```python
from build123d import *

# Parameters (mm, degrees)
ESQUISSE1_R             = 2
ESQUISSE1_R_2           = 1.5
BOSS_EXTRU_1_DEPTH      = 3
ESQUISSE3_R             = 7.5
BOSS_EXTRU_2_DEPTH      = 6
ESQUISSE4_R             = 3.875
ENL_V_MAT_EXTRU_1_DEPTH = 1
ESQUISSE5_R             = 2.375
ENL_V_MAT_EXTRU_2_DEPTH = 4


with BuildPart() as part:
    # Esquisse1 → Boss.-Extru.1 (new body)
    with BuildSketch(Plane.XY):
        Polygon((0, 50), (-100, 50), (-100, 0), (-61.381557247, 0), (-61.381557247, -45.5212086), (-25, -45.5212086), (-25, -80), (25, -80), (25, -45.5212086), (61.381557247, -45.5212086), (61.381557247, 0), (100, 0), (100, 50), align=None)
        with Locations((0, 20)):
            Circle(ESQUISSE1_R, mode=Mode.SUBTRACT)
        with Locations((0, -20)):
            Circle(ESQUISSE1_R, mode=Mode.SUBTRACT)
        with Locations((0, 40)):
            Circle(ESQUISSE1_R, mode=Mode.SUBTRACT)
        with Locations((-20, -55)):
            Circle(ESQUISSE1_R_2, mode=Mode.SUBTRACT)
        with Locations((20, -55)):
            Circle(ESQUISSE1_R_2, mode=Mode.SUBTRACT)
        with Locations((20, -75)):
            Circle(ESQUISSE1_R_2, mode=Mode.SUBTRACT)
        with Locations((-20, -75)):
            Circle(ESQUISSE1_R_2, mode=Mode.SUBTRACT)
        with Locations((-95, 45)):
            Circle(ESQUISSE1_R_2, mode=Mode.SUBTRACT)
        with Locations((-75, 45)):
            Circle(ESQUISSE1_R_2, mode=Mode.SUBTRACT)
        with Locations((-75, 5)):
            Circle(ESQUISSE1_R_2, mode=Mode.SUBTRACT)
        with Locations((-95, 5)):
            Circle(ESQUISSE1_R_2, mode=Mode.SUBTRACT)
        with Locations((75, 5)):
            Circle(ESQUISSE1_R_2, mode=Mode.SUBTRACT)
        with Locations((95, 5)):
            Circle(ESQUISSE1_R_2, mode=Mode.SUBTRACT)
        with Locations((75, 45)):
            Circle(ESQUISSE1_R_2, mode=Mode.SUBTRACT)
        with Locations((95, 45)):
            Circle(ESQUISSE1_R_2, mode=Mode.SUBTRACT)
        with Locations((56.381557247, -40.5212086)):
            Circle(ESQUISSE1_R, mode=Mode.SUBTRACT)
        with Locations((-56.381557247, -40.5212086)):
            Circle(ESQUISSE1_R, mode=Mode.SUBTRACT)
    extrude(amount=BOSS_EXTRU_1_DEPTH)

    # Esquisse3 → Boss.-Extru.2 (add)
    with BuildSketch(Plane(origin=(0, 0, 0), x_dir=(-1, 0, 0), z_dir=(0, 0, -1))):
        with Locations((0, 20)):
            Circle(ESQUISSE3_R)
        with Locations((56.381557247, -40.5212086)):
            Circle(ESQUISSE3_R)
    extrude(amount=-BOSS_EXTRU_2_DEPTH)

    # Esquisse4 → Enlèv. mat.-Extru.1 (cut)
    with BuildSketch(Plane.XY.offset(6)):
        with Locations((-56.381557247, -40.5212086)):
            Circle(ESQUISSE4_R)
        with Locations((0, 20)):
            Circle(ESQUISSE4_R)
    extrude(amount=-ENL_V_MAT_EXTRU_1_DEPTH, mode=Mode.SUBTRACT)

    # Esquisse5 → Enlèv. mat.-Extru.2 (cut)
    with BuildSketch(Plane.XY.offset(5)):
        with Locations((-56.381557247, -40.5212086)):
            Circle(ESQUISSE5_R)
        with Locations((0, 20)):
            Circle(ESQUISSE5_R)
    extrude(amount=-ENL_V_MAT_EXTRU_2_DEPTH, mode=Mode.SUBTRACT)


solid = part.part
```
Verification items for the finished model (mm, model axes). A direction names the side the tool comes from. Give positions to 0.01 mm unless a question says otherwise; leave off trailing zeros. Order: outer loops, then holes, each group sorted by start corner. A loop starts at its lowest first (then second) coordinate and runs counter-clockwise, first axis right, second up. Notation, with made-up numbers: M 58.25,33 L 84.25,33 A20 ccw 84.25,48 Z; hole C 24,-34.5 d5. An arc over 180 degrees is marked long. Answer in a Markdown table with one row per item. Add a question column.
Item 1: Section check D-D, the plane y = -20. Enter the section's corners in (x, z).
Item 2: Section check B-B, the plane y = 20. Enter the section's corners in (x, z) (3 decimals).
Item 3: Gauge pin test, flat ends, axial feed: pin 1 (2.5 mm diameter, centred on y = -58, z = 1.5, fed in from -X); pin 2 (4 mm diameter, centred on x = 0, y = 20, fed in from +Z); pin 3 (4 mm diameter, centred on x = -20, y = -55, fed in from +Z); pin 4 (3 mm diameter, centred on x = 0, y = -20, fed in from +Z). Record the tip position at first contact, or that the pin passes through.
Item 4: Section check A-A, the plane y = 40. Enter the section's corners in (x, z).
Item 5: Mould release check, pull along Y, two halves, no side actions. Record for faces 3 (the cylindrical face through (0.976, 27.436, 4.479)), 4 (the cylindrical face through (54.907, -39.17, 1.479)), 5 (the cylindrical face through (0, 38, 1)), 6 (the flat face through (-3, 17, 6)): released by +Y, released by -Y, zero draft, split by the parting line, or undercut.
Item 6: Scan lines: probe 1 along Y at (x, z) = (-95, 1.45); probe 2 along Y at (x, z) = (20, 1.9); probe 3 along X at (y, z) = (4, 0.55). Record each from-to range of solid material in increasing order. Write a range as from..to.
Item 7: Section check C-C, the plane x = 46.5. Enter the section's corners in (y, z).
Item 8: Tool access check on faces 1 (the cylindrical face through (0, -18, 1)), 2 (the flat face through (0, 20, 1)). Record the directions out of +Z, -Z, +X, -X, +Y, -Y that give a thin tool (end or side, any length) a straight path to the whole face; none if there is none.
Filled sheet:
| question | item | result |
|---|---|---|
| 1 | outline | M -61.38,0 L -2,0 L -2,3 L -61.38,3 Z; M 2,0 L 61.38,0 L 61.38,3 L 2,3 Z |
| 2 | outline | M -100,0 L 100,0 L 100,3 L 7.5,3 L 7.5,6 L 3.875,6 L 3.875,5 L 2.375,5 L 2.375,1 L -2.375,1 L -2.375,5 L -3.875,5 L -3.875,6 L -7.5,6 L -7.5,3 L -100,3 Z |
| 3 | pin 1 | stops at x = -25 |
| 3 | pin 2 | stops at z = 1 |
| 3 | pin 3 | stops at z = 3 |
| 3 | pin 4 | passes through |
| 4 | outline | M -100,0 L -2,0 L -2,3 L -100,3 Z; M 2,0 L 100,0 L 100,3 L 2,3 Z |
| 5 | face 3 | split by the parting line |
| 5 | face 4 | undercut |
| 5 | face 5 | undercut |
| 5 | face 6 | zero draft |
| 6 | probe 1 | y = 0..3.5, 6.5..43.5, 46.5..50 |
| 6 | probe 2 | y = -80..-76.5, -73.5..-56.5, -53.5..50 |
| 6 | probe 3 | x = -100..-96.12, -93.88..-76.12, -73.88..73.88, 76.12..93.88, 96.12..100 |
| 7 | outline | M -45.52,0 L 50,0 L 50,3 L -45.52,3 Z |
| 8 | face 1 | +Z, -Z |
| 8 | face 2 | +Z |
